Read the model definition and answer for the solid it produces. Units are mm, in the model's axes. Round coordinates to 2 decimals unless told otherwise and drop trailing zeros. Order: outer loops, then holes, each group sorted by start corner. A loop starts at its lowest first (then second) coordinate and runs counter-clockwise, first axis right, second up. Notation, with made-up numbers: (60, -26.75) - (103, -26.75) arc R22 cw to (103, 7.25) - close; hole circle Ø10 at (4.25, -30). An arc over 180 degrees is marked (long way). Answer as a JSON object with one key per item and string values. Group by question number.
Q1. Given pin 1 Ø6 at (x, z) = (9, -181.5) entering from -Y; pin 2 Ø1 at (x, z) = (7, -223.5) entering from +Y; pin 3 Ø2 at (x, y) = (-7.5, -1) entering from +Z, each flat-ended and moving along its own axis, determine where each tip first touches the part or whether it passes through.
Q2. A cutting plane is placed at C-C on y = 21. Determine the outline of the cut face in (x, z).
Q3. A cutting plane is placed at B-B on x = 4.75. Determine the outline of the cut face in (y, z) (3 decimals), and give its area (3 significant figures).
Q4. Consider line 1 (Z direction, x = -4.5, y = 0); line 2 (Y direction, x = 6, z = -388.5); line 3 (Z direction, x = -10, y = 22). Determine where each line is inside the solid, lowest interval first.
Q5. A cutting plane is placed at A-A on z = -412. Determine the outline of the cut face in (x, y).
```python
from build123d import *

# Parameters (mm, degrees)
SKETCH1_R           = 2.5527
BOSS_EXTRUDE1_DEPTH = 12.7
SKETCH3_R           = 25.4
BOSS_EXTRUDE2_DEPTH = 6.35
SKETCH4_R           = 2.5527
CUT_EXTRUDE1_DEPTH  = 459.301104624
FILLET1_R           = 6.35


with BuildPart() as part:
    # Sketch1 → Boss-Extrude1 (new, symmetric)
    with BuildSketch(Plane(origin=(0, 0, 0), x_dir=(0, 0, -1), z_dir=(1, 0, 0))):
        with BuildLine():
            Line((0, 12.7), (457.2, 12.7))
            Line((457.2, 12.7), (457.2, -12.7))
            Line((457.2, -12.7), (0, -12.7))
            ThreePointArc((0, -12.7), (-12.7, 0), (0, 12.7))
        make_face()
        with Locations((3.175, 5.499261314)):
            Circle(SKETCH1_R, mode=Mode.SUBTRACT)
        with Locations((-6.35, 0)):
            Circle(SKETCH1_R, mode=Mode.SUBTRACT)
        with Locations((3.175, -5.499261314)):
            Circle(SKETCH1_R, mode=Mode.SUBTRACT)
    extrude(amount=BOSS_EXTRUDE1_DEPTH, both=True)

    # Sketch3 → Boss-Extrude2 (add)
    with BuildSketch(Plane.ZY.offset(12.7)):
        Circle(SKETCH3_R)
    extrude(amount=-BOSS_EXTRUDE2_DEPTH)

    # Sketch4 → Cut-Extrude1 (cut, through all)
    with BuildSketch(Plane(origin=(-6.35, 0, 0), x_dir=(0, 0, -1), z_dir=(1, 0, 0))):
        with Locations((3.175, 5.499261314)):
            Circle(SKETCH4_R)
        with Locations((3.175, -5.499261314)):
            Circle(SKETCH4_R)
        with Locations((-6.35, 0)):
            Circle(SKETCH4_R)
    extrude(amount=-CUT_EXTRUDE1_DEPTH, mode=Mode.SUBTRACT)

    # Fillet1
    fillet1_edges = [part.edges().sort_by_distance(p)[0] for p in [
        (-9.525, 12.7, -21.997045256),
        (-9.525, -12.7, -21.997045256),
    ]]
    fillet(fillet1_edges, radius=FILLET1_R)


solid = part.part
```
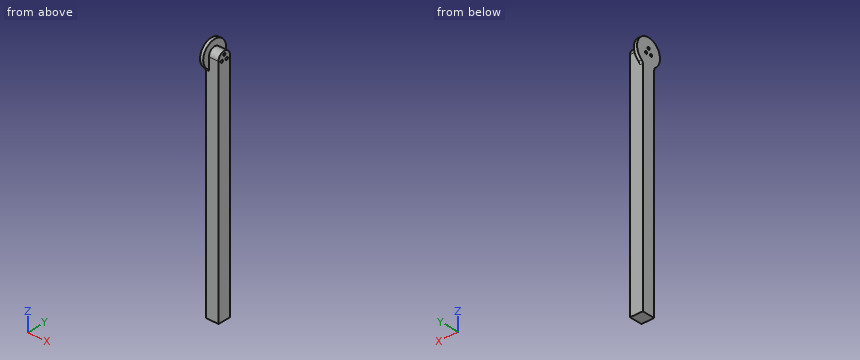
Result set:
{
 "1": {"pin 1": "stops at y = -12.7", "pin 2": "stops at y = 12.7", "pin 3": "stops at z = 25.4"},
 "2": {"outline": "(-12.7, -14.29) - (-6.35, -14.29) - (-6.35, 14.29) - (-12.7, 14.29) - close"},
 "3": {"outline": "(-12.7, -457.2) - (12.7, -457.2) - (12.7, 0) arc R12.7 ccw to (-12.7, 0) - close; hole circle Ø5.105 at (-5.499, -3.175); hole circle Ø5.105 at (0, 6.35); hole circle Ø5.105 at (5.499, -3.175)", "area": "11,800 mm²"},
 "4": {"line 1": "z = -457.2 to 3.8, 8.9 to 12.7", "line 2": "y = -12.7 to 12.7", "line 3": "z = -12.69 to 12.69"},
 "5": {"outline": "(-12.7, -12.7) - (12.7, -12.7) - (12.7, 12.7) - (-12.7, 12.7) - close"}
}
